The model under review builds one solid part; all positions refer to its coordinate system, in mm. Round coordinates to 2 decimals unless told otherwise and drop trailing zeros. Write each loop counter-clockwise with the first axis right and the second up, starting at its lowest first coordinate (ties: lowest second). Pieces come first, ordered by that corner, then holes. Notation, with made-up numbers: M 3.25,55.5 L 12.25,55.5 A9 cw 12.25,65.5 Z; hole C 54,0.25 d10. An arc over 180 degrees is marked long. One line per item, written item: value. Start each with the question number.
1) Wall thickness on probe 1 along Z at (x, y) = (-1, 2.15); probe 2 along X at (y, z) = (1, -271.5); probe 3 along X at (y, z) = (2.25, -191.5): over which ranges is each line inside the solid? List them lowest first.
2) Take a section at A-A, the plane y = 0.5. State how many separate pieces and enclosed holes the cut face has, and give its area (3 significant figures).
3) Take a section at B-B, the plane x = 242. Write out the cut boundary in (y, z), and give its area (3 significant figures).
4) Take a section at C-C, the plane z = -82.5. Write out the cut boundary in (x, y).
5) For P1, Ø1.5, axis at x = 158, y = 1, coming from the -Z side; P2, Ø1, axis at y = 1.5, z = -18.5, coming from the -X side; P3, Ø1.8, axis at x = 81.35, z = -59.09, coming from the -Y side; P4, Ø1.5, axis at y = 1.5, z = -123, coming from the -X side, all flat-tipped, find the tip position at first contact; note any pin that passes through.
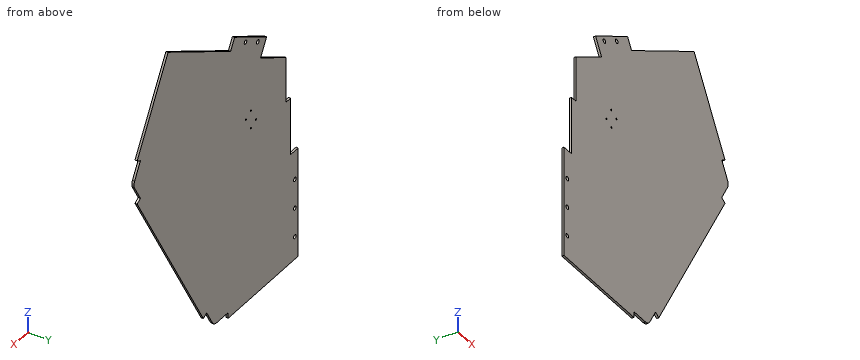
Autodesk Inventor part; units mm, degrees
ref_plane "YZ Plane" through (0, 0, 0) normal (1, 0, 0) x (0, 1, 0)
ref_plane "XZ Plane" through (0, 0, 0) normal (0, 1, 0) x (-1, 0, 0)
ref_plane "XY Plane" through (0, 0, 0) normal (0, 0, 1) x (1, 0, 0)
sketch "Sketch1" plane through (0, 0, 0) normal (0, 1, 0) x (-1, 0, 0)
  line L0 (349.8743, 0) -> (258.4057, -158.4282)
  line L1 (174.9371, -303) -> (-174.9371, -303)
  line L2 (-174.9371, -303) -> (-349.8743, 0)
  line L3 (-349.8743, 0) -> (-174.9371, 303)
  line L4 (-174.9371, 303) -> (174.9371, 303)
  line L5 (258.4057, 158.4282) -> (349.8743, 0)
  line L6 (0, 0) -> (-8, 0)
  line L7 (-8, 0) -> (-8, -303)
  line L8 (-8, -303) -> (8, -303)
  line L9 (8, -303) -> (8, 0)
  line L10 (8, 0) -> (-8, 0)
  circle A0 centre (0, 0) radius 2.5
  line L11 (258.4057, 158.4282) -> (-4, 6.9282)
  line L12 (4, -6.9282) -> (266.4057, 144.5718)
  line L13 (-4, 6.9282) -> (4, -6.9282)
  line L14 (-266.4057, 144.5718) -> (-4, -6.9282)
  line L15 (4, 6.9282) -> (-258.4057, 158.4282)
  line L16 (-4, -6.9282) -> (4, 6.9282)
  line L17 (8, -4.6188) -> (8, -151.5)
  line L18 (8, -151.5) -> (-8, -151.5)
  line L19 (-8, -151.5) -> (-8, -303)
  line L20 (-8, -4.6188) -> (-4, -6.9282)
  line L21 (4, -6.9282) -> (-4, -6.9282)
  line L22 (-266.4057, 144.5718) -> (-258.4057, 158.4282)
  line L23 (-127.2028, 82.6782) -> (-135.2028, 68.8218)
  line L24 (-135.2028, 68.8218) -> (-8, -4.6188)
  line L25 (-266.4057, 144.5718) -> (-349.8743, 0)
  line L26 (-174.9371, -303) -> (-349.8743, 0)
  line L27 (-174.9371, -303) -> (-8, -303)
  line L28 (0, 9.2376) -> (8, 0)
  dimension "d0" = 303
  dimension "d1" = 303
  dimension "d2" = 8
  dimension "d3" = 16
  dimension "d4" = 5
  dimension "d7" = 360
extrude "Extrusion1" add sketch "Sketch1" along normal blind 3 contours L1 L7 L18 L9 | L1 L2 L3 L14 L7 | L18 L7 L14 L21 L12 L9 | L12 L13 A0 L10 L9 | L14 L23 L15 L11 L13 A0 L6 L7 | L7 L6 A0 L16 L14 | L10 A0 L16 L28 | L21 L16 A0 L13 | L3 L15 L23 L14 | A0 L13 L10 | L10 L16 A0 | L28 L15 L16 | L16 A0 L13 L11 L28 | A0 L16 L13 | A0 L13 L6 | L6 L16 A0 | L13 A0 L16
sketch "Sketch2" plane through (0, 3, 0) normal (0, 1, 0) x (1, 0, 0)
  line L0 (-8, 303) -> (-8, 0)
  line L1 (-8, 0) -> (-8, 151.5)
  line L2 (-8, 151.5) -> (8, 151.5)
  line L3 (8, 151.5) -> (8, 0)
  line L4 (8, 0) -> (-8, 0)
  line L5 (0, -9.2376) -> (258.4057, -158.4282)
  line L6 (258.4057, -158.4282) -> (126.3368, -82.1782)
  line L7 (126.3368, -82.1782) -> (134.8368, -67.4558)
  line L8 (134.8368, -67.4558) -> (266.9057, -143.7058)
  line L9 (266.9057, -143.7058) -> (258.4057, -158.4282)
  point P0 (0, 0)
  dimension "d11" = 151.5
  dimension "d12" = 16
  dimension "d13" = 152.5
  dimension "d14" = 17
extrude "Extrusion2" cut sketch "Sketch2" against normal blind 3
sketch "Sketch3" plane through (0, 3, 0) normal (0, 1, 0) x (1, 0, 0)
  line L0 (174.9371, 303) -> (-8, 303)
  line L1 (174.9371, 303) -> (139.9371, 303)
  line L2 (139.9371, 303) -> (139.9371, 295)
  line L3 (139.9371, 295) -> (174.9371, 295)
  line L4 (174.9371, 295) -> (174.9371, 303)
  line L5 (349.8743, 0) -> (174.9371, 303)
  line L6 (174.9371, 303) -> (192.4371, 272.6891)
  line L7 (192.4371, 272.6891) -> (185.5089, 268.6891)
  line L8 (185.5089, 268.6891) -> (168.0089, 299)
  line L9 (168.0089, 299) -> (174.9371, 303)
  line L10 (349.8743, 0) -> (332.3743, 30.3109)
  line L11 (332.3743, 30.3109) -> (325.4461, 26.3109)
  line L12 (325.4461, 26.3109) -> (342.9461, -4)
  line L13 (342.9461, -4) -> (349.8743, 0)
  line L14 (349.8743, 0) -> (332.3743, -30.3109)
  line L15 (332.3743, -30.3109) -> (325.4461, -26.3109)
  line L16 (325.4461, -26.3109) -> (342.9461, 4)
  line L17 (342.9461, 4) -> (349.8743, 0)
  line L18 (349.8743, 0) -> (266.9057, -143.7058)
  line L19 (349.8743, 0) -> (384.8743, 0) construction
  point P0 (0, 0)
  dimension "d17" = 35
  dimension "d18" = 8
  dimension "d19" = 35
  dimension "d20" = 8
  dimension "d21" = 35
  dimension "d22" = 8
  dimension "d23" = 35
  dimension "d24" = 120
  dimension "d25" = 8
extrude "Extrusion3" cut sketch "Sketch3" against normal blind 3
sketch "Sketch4" plane through (0, 3, 0) normal (0, 1, 0) x (1, 0, 0)
  line L0 (-54.0368, 51.4054) -> (71.5368, -21.0946)
  line L1 (71.5368, -21.0946) -> (54.0368, -51.4054)
  line L2 (54.0368, -51.4054) -> (-71.5368, 21.0946)
  line L3 (-71.5368, 21.0946) -> (-54.0368, 51.4054)
  line L4 (-54.0368, 51.4054) -> (54.0368, -51.4054) construction
  line L5 (71.5368, -21.0946) -> (-71.5368, 21.0946) construction
  line L6 (-54.0368, 51.4054) -> (90.9632, 51.4054) construction
  line L7 (-17.5, -72.5) -> (-17.5, 72.5)
  line L8 (-17.5, 72.5) -> (17.5, 72.5)
  line L9 (17.5, 72.5) -> (17.5, -72.5)
  line L10 (17.5, -72.5) -> (-17.5, -72.5)
  line L11 (-17.5, -72.5) -> (17.5, 72.5) construction
  line L12 (-17.5, 72.5) -> (17.5, -72.5) construction
  line L13 (-8, 0) -> (8, 0)
  line L14 (-17.5, -72.5) -> (127.5, -72.5) construction
  point P0 (0, 0)
  dimension "d28" = 145
  dimension "d29" = 30
  dimension "d30" = 35
  dimension "d31" = 145
  dimension "d32" = 90
  dimension "d33" = 35
extrude "Extrusion4" cut sketch "Sketch4" against normal blind 3
sketch "Sketch5" plane through (0, 3, 0) normal (0, 1, 0) x (1, 0, 0)
  line L0 (-1, 151.5) -> (-1, 191.5)
  circle A0 centre (-1, 191.5) radius 2.75
  circle A1 centre (-1, 231.5) radius 2.75
  circle A2 centre (-1, 271.5) radius 2.75
  circle A3 centre (0, 0) radius 0.5
  line L1 (126.3368, -82.1782) -> (134.8368, -67.4558)
  line L2 (126.3368, -82.1782) -> (129.3368, -76.9821)
  line L3 (129.3368, -76.9821) -> (103.3561, -61.9821)
  line L4 (103.3561, -61.9821) -> (77.3753, -46.9821)
  circle A4 centre (103.3561, -61.9821) radius 2.75
  circle A5 centre (77.3753, -46.9821) radius 2.75
  line L5 (-8, 303) -> (-8, 151.5)
  dimension "d36" = 40
  dimension "d37" = 5.5
  dimension "d40" = 40
  dimension "d45" = 1
  dimension "d46" = 6
  dimension "d47" = 30
  dimension "d48" = 30
  dimension "d49" = 5.5
  dimension "d50" = 5.5
  dimension "d53" = 7
extrude "Extrusion5" cut sketch "Sketch5" against normal blind 3 contours A0 | A1 | A2 | A4 L4 L3 | A5 | L3 L4 A4
sketch "Sketch6" plane through (0, 3, 0) normal (0, 1, 0) x (1, 0, 0)
  line L0 (-8, 303) -> (-8, 151.5)
  line L1 (-8, 303) -> (344, 303)
  line L2 (344, 303) -> (344, -147)
  line L3 (344, -147) -> (-8, -147)
  line L4 (-8, -147) -> (-8, 303)
  point P0 (0, 0)
  dimension "d54" = 352
  dimension "d55" = 450
sketch "Sketch7" plane through (0, 3, 0) normal (0, 1, 0) x (1, 0, 0)
  line L0 (0, 0) -> (86.6025, 50)
  line L1 (0, 0) -> (100, 0) construction
  line L2 (86.6025, 50) -> (91.8525, 40.9067)
  circle A0 centre (91.8525, 40.9067) radius 1.1
  line L3 (86.6025, 50) -> (89.2006, 51.5)
  line L4 (86.6025, 50) -> (89.6025, 50) construction
  circle A1 centre (81.3525, 59.0933) radius 1.1
  circle A2 centre (102.6779, 47.1567) radius 1.1
  circle A3 centre (92.1779, 65.3433) radius 1.1
  dimension "d56" = 100
  dimension "d57" = 30
  dimension "d58" = 10.5
  dimension "d59" = 90
  dimension "d60" = 2.2
  dimension "d61" = 3
  dimension "d62" = 30
  dimension "d65" = 21
  dimension "d68" = 12.5
extrude "Extrusion6" cut sketch "Sketch7" against normal blind 5
fillet "Fillet1" radius 10 2 edges at (340.6367, 1.5, 0) (170.3183, 1.5, -295)
properties part number "Acrylic_bottom_camera"
Checked values:
1. probe 1: z = -303 to -274.25, -268.75 to -234.25, -228.75 to -194.25, -188.75 to -151.5
1. probe 2: x = -8 to -3.75, 1.75 to 183.89, 190.38 to 193.12
1. probe 3: x = -8 to -3.75, 1.75 to 239.31
2. separate pieces: 1
2. enclosed holes: 9
2. area: 102,000 mm2
3. outline: M 0,-186.84 L 3,-186.84 L 3,129.33 L 0,129.33 Z
3. area: 949 mm2
4. outline: M 8,0 L 302.24,0 L 302.24,3 L 8,3 Z
5. P1: stops at z = -295
5. P2: stops at x = 17.5
5. P3: passes through
5. P4: stops at x = 8
